Autodesk Inventor part; units mm, degrees
ref_plane "YZ Plane" through (0, 0, 0) normal (1, 0, 0) x (0, 1, 0)
ref_plane "XZ Plane" through (0, 0, 0) normal (0, 1, 0) x (-1, 0, 0)
ref_plane "XY Plane" through (0, 0, 0) normal (0, 0, 1) x (1, 0, 0)
sketch "Sketch1" plane through (0, 0, 0) normal (0, 0, 1) x (1, 0, 0)
  point P0 (0, 0)
sketch "Sketch2" plane through (0, 0, 0) normal (0, 0, 1) x (1, 0, 0)
  line L0 (0, 0) -> (5, 0)
  line L1 (5, 0) -> (5, 5)
  line L2 (5, 5) -> (0, 5)
  line L3 (0, 5) -> (0, 0)
  line L4 (5, 5) -> (105, 5)
  line L5 (105, 5) -> (105, 55)
  line L6 (105, 55) -> (5, 55)
  line L7 (5, 55) -> (5, 5)
  line L8 (105, 55) -> (110, 55)
  line L9 (110, 55) -> (110, 60)
  line L10 (110, 60) -> (105, 60)
  line L11 (105, 60) -> (105, 55)
  line L12 (100, 60) -> (95, 60)
  line L13 (100, 55) -> (100, 60)
  line L14 (95, 60) -> (95, 55)
  line L15 (90, 60) -> (85, 60)
  line L16 (90, 55) -> (90, 60)
  line L17 (85, 60) -> (85, 55)
  line L18 (80, 60) -> (75, 60)
  line L19 (80, 55) -> (80, 60)
  line L20 (75, 60) -> (75, 55)
  line L21 (70, 60) -> (65, 60)
  line L22 (70, 55) -> (70, 60)
  line L23 (65, 60) -> (65, 55)
  line L24 (60, 60) -> (55, 60)
  line L25 (60, 55) -> (60, 60)
  line L26 (55, 60) -> (55, 55)
  line L27 (50, 60) -> (45, 60)
  line L28 (50, 55) -> (50, 60)
  line L29 (45, 60) -> (45, 55)
  line L30 (40, 60) -> (35, 60)
  line L31 (40, 55) -> (40, 60)
  line L32 (35, 60) -> (35, 55)
  line L33 (30, 60) -> (25, 60)
  line L34 (30, 55) -> (30, 60)
  line L35 (25, 60) -> (25, 55)
  line L36 (20, 60) -> (15, 60)
  line L37 (20, 55) -> (20, 60)
  line L38 (15, 60) -> (15, 55)
  line L39 (10, 60) -> (5, 60)
  line L40 (10, 55) -> (10, 60)
  line L41 (5, 60) -> (5, 55)
  line L42 (105, 50) -> (105, 45)
  line L43 (110, 45) -> (110, 50)
  line L44 (110, 50) -> (105, 50)
  line L45 (105, 45) -> (110, 45)
  line L46 (105, 40) -> (105, 35)
  line L47 (110, 35) -> (110, 40)
  line L48 (110, 40) -> (105, 40)
  line L49 (105, 35) -> (110, 35)
  line L50 (105, 30) -> (105, 25)
  line L51 (110, 25) -> (110, 30)
  line L52 (110, 30) -> (105, 30)
  line L53 (105, 25) -> (110, 25)
  line L54 (105, 20) -> (105, 15)
  line L55 (110, 15) -> (110, 20)
  line L56 (110, 20) -> (105, 20)
  line L57 (105, 15) -> (110, 15)
  line L58 (105, 10) -> (105, 5)
  line L59 (110, 5) -> (110, 10)
  line L60 (110, 10) -> (105, 10)
  line L61 (105, 5) -> (110, 5)
  line L62 (0, 10) -> (5, 10)
  line L63 (5, 10) -> (5, 15)
  line L64 (5, 15) -> (0, 15)
  line L65 (0, 15) -> (0, 10)
  line L66 (0, 20) -> (5, 20)
  line L67 (5, 20) -> (5, 25)
  line L68 (5, 25) -> (0, 25)
  line L69 (0, 25) -> (0, 20)
  line L70 (0, 30) -> (5, 30)
  line L71 (5, 30) -> (5, 35)
  line L72 (5, 35) -> (0, 35)
  line L73 (0, 35) -> (0, 30)
  line L74 (0, 40) -> (5, 40)
  line L75 (5, 40) -> (5, 45)
  line L76 (5, 45) -> (0, 45)
  line L77 (0, 45) -> (0, 40)
  line L78 (0, 50) -> (5, 50)
  line L79 (5, 50) -> (5, 55)
  line L80 (5, 55) -> (0, 55)
  line L81 (0, 55) -> (0, 50)
  line L82 (15, 5) -> (10, 5)
  line L83 (10, 0) -> (15, 0)
  line L84 (15, 0) -> (15, 5)
  line L85 (10, 5) -> (10, 0)
  line L86 (25, 5) -> (20, 5)
  line L87 (20, 0) -> (25, 0)
  line L88 (25, 0) -> (25, 5)
  line L89 (20, 5) -> (20, 0)
  line L90 (35, 5) -> (30, 5)
  line L91 (30, 0) -> (35, 0)
  line L92 (35, 0) -> (35, 5)
  line L93 (30, 5) -> (30, 0)
  line L94 (45, 5) -> (40, 5)
  line L95 (40, 0) -> (45, 0)
  line L96 (45, 0) -> (45, 5)
  line L97 (40, 5) -> (40, 0)
  line L98 (55, 5) -> (50, 5)
  line L99 (50, 0) -> (55, 0)
  line L100 (55, 0) -> (55, 5)
  line L101 (50, 5) -> (50, 0)
  line L102 (65, 5) -> (60, 5)
  line L103 (60, 0) -> (65, 0)
  line L104 (65, 0) -> (65, 5)
  line L105 (60, 5) -> (60, 0)
  line L106 (75, 5) -> (70, 5)
  line L107 (70, 0) -> (75, 0)
  line L108 (75, 0) -> (75, 5)
  line L109 (70, 5) -> (70, 0)
  line L110 (85, 5) -> (80, 5)
  line L111 (80, 0) -> (85, 0)
  line L112 (85, 0) -> (85, 5)
  line L113 (80, 5) -> (80, 0)
  line L114 (95, 5) -> (90, 5)
  line L115 (90, 0) -> (95, 0)
  line L116 (95, 0) -> (95, 5)
  line L117 (90, 5) -> (90, 0)
  line L118 (105, 5) -> (100, 5)
  line L119 (100, 0) -> (105, 0)
  line L120 (105, 0) -> (105, 5)
  line L121 (100, 5) -> (100, 0)
  dimension "d11" = 10
  dimension "d0" = 5
  dimension "d1" = 5
  dimension "d4" = 5
  dimension "d5" = 5
  dimension "d8" = 10
  dimension "d15" = 10
  dimension "d22" = 10
  dimension "d29" = 10
sketch "Sketch3" plane through (0, 0, 0) normal (0, 0, 1) x (1, 0, 0)
  point P0 (0, 0)
extrude "Extrusion1" add sketch "Sketch2" along normal blind 5 contours L7 L6 L5 L4 | L62 L65 L64 L7 | L66 L69 L68 L7 | L70 L73 L72 L7 | L74 L77 L76 L7 | L78 L81 L80 L7 | L41 L39 L40 L6 | L38 L36 L37 L6 | L35 L33 L34 L6 | L32 L30 L31 L6 | L29 L27 L28 L6 | L5 L60 L59 L61 | L26 L24 L25 L6 | L5 L56 L55 L57 | L23 L21 L22 L6 | L5 L52 L51 L53 | L20 L18 L19 L6 | L5 L48 L47 L49 | L17 L15 L16 L6 | L5 L44 L43 L45 | L14 L12 L13 L6
properties part number "frontbackside"
Check sheet for the modelled part. Datum: model origin and axes. Units: mm. A direction names the side the tool comes from. Give positions to 0.01 mm unless a question says otherwise; leave off trailing zeros. Loops run counter-clockwise (first coordinate to the right, second up) from the corner with the lowest first, then second, coordinate; pieces in that order, holes last. Notation, with made-up numbers: M 13.25,63.5 L 50.25,63.5 A29 ccw 50.25,91.5 Z; hole C 62,56 d11. An arc over 180 degrees is marked long. Return JSON: item names as keys, results as strings. Group by question number.
1. Thickness scan on L1, parallel to Y at x = 24, z = 2.95; L2, parallel to X at y = 54, z = 3.5; L3, parallel to X at y = 8, z = 2.3. Record the ranges inside material, lowest first.
2. Mould release check, pull along X, two halves, no side actions. Record for faces 5 (the flat face through (0, 43, 2)), 6 (the flat face through (73, 55, 2)), 7 (the flat face through (110, 27, 2)): released by +X, released by -X, zero draft, split by the parting line, or undercut.
3. Cross-section at A-A on y = 54. Record the boundary of the cut face in (x, z).
4. Cross-section at B-B on x = 63.5. Record the boundary of the cut face in (y, z), plus the area to 3 significant figures.
5. Go/stop test with flat-tipped pins: pin 1 (2.5 mm diameter, centred on y = 58, z = 2.5, fed in from -X); pin 2 (1.5 mm diameter, centred on y = 57, z = 3.5, fed in from +X); pin 3 (1.5 mm diameter, centred on x = 3.5, z = 3, fed in from -Y). Record where each tip stops, or that it passes through.
6. Tool access check on faces 1 (the flat face through (35, 58, 2)), 2 (the flat face through (2, 10, 2)), 3 (the flat face through (108, 40, 2)), 4 (the flat face through (3, 25, 2)). Record the directions out of +Z, -Z, +X, -X, +Y, -Y that give a thin tool (end or side, any length) a straight path to the whole face; none if there is none.
Return value:
{
 "1": {"L1": "5 to 55", "L2": "0 to 105", "L3": "5 to 110"},
 "2": {"face 5": "released by -X", "face 6": "undercut", "face 7": "released by +X"},
 "3": {"outline": "M 0,0 L 105,0 L 105,5 L 0,5 Z"},
 "4": {"outline": "M 5,0 L 55,0 L 55,5 L 5,5 Z", "area": "250 mm^2"},
 "5": {"pin 1": "x = 5", "pin 2": "x = 100", "pin 3": "y = 10"},
 "6": {"face 1": "+Z, -Z, +Y", "face 2": "+Z, -Z, -X, -Y", "face 3": "+Z, -Z, +X", "face 4": "+Z, -Z, -X"}
}
